```python
from build123d import *

# Parameters (mm, degrees)
F0_R     = 1.651
F1_DEPTH = 3.175
F2_R     = 1.651
F3_DEPTH = 25.4


with BuildPart() as f1:
    # F0 (on Front) → F1 (new body)
    with BuildSketch(Plane.XZ):
        with BuildLine():
            Line((65.389104, 5.08), (65.389104, 0))
            Line((65.389104, 0), (111.109104, 0))
            Line((111.109104, 0), (134.019904, 0))
            Line((134.019904, 0), (139.049104, 0))
            Line((139.049104, 0), (139.477193, 0))
            ThreePointArc((139.477193, 0), (148.009982, 3.664074), (152.4, 11.847085))
            Line((152.4, 11.847085), (152.4, 30.797511))
            ThreePointArc((152.4, 30.797511), (134.859224, 59.672781), (105.392106, 76.2))
            Line((105.392106, 76.2), (37.521991, 76.2))
            Line((37.521991, 76.2), (12.7, 76.2))
            Line((12.7, 76.2), (12.7, 71.12))
            Line((12.7, 71.12), (0, 71.12))
            Line((0, 71.12), (0, 76.2))
            Line((0, 76.2), (-25.4, 76.2))
            Line((-25.4, 76.2), (-25.4, 71.12))
            Line((-25.4, 71.12), (-38.1, 71.12))
            Line((-38.1, 71.12), (-38.1, 76.2))
            Line((-38.1, 76.2), (-50.8, 76.2))
            Line((-50.8, 76.2), (-50.8, 0))
            Line((-50.8, 0), (-19.015096, 0))
            Line((-19.015096, 0), (-19.015096, 5.08))
            Line((-19.015096, 5.08), (65.389104, 5.08))
        make_face()
        with Locations((-36.449, 11.697368)):
            Circle(F0_R, mode=Mode.SUBTRACT)
        with Locations((-12.364374, 17.884336)):
            Circle(F0_R, mode=Mode.SUBTRACT)
        with Locations((16.566699, 25.316282)):
            Circle(F0_R, mode=Mode.SUBTRACT)
        with Locations((40.651325, 31.503251)):
            Circle(F0_R, mode=Mode.SUBTRACT)
        with Locations((79.176886, 41.399872)):
            Circle(F0_R, mode=Mode.SUBTRACT)
        with Locations((104.294765, 47.852268)):
            Circle(F0_R, mode=Mode.SUBTRACT)
    extrude(amount=F1_DEPTH)

    # F2 (on face) → F3 (cut)
    with BuildSketch(Plane.XZ.offset(3.175)):
        with Locations((148.009982, 9.237001)):
            Circle(F2_R)
    extrude(amount=-F3_DEPTH, mode=Mode.SUBTRACT)


solid = f1.part
```
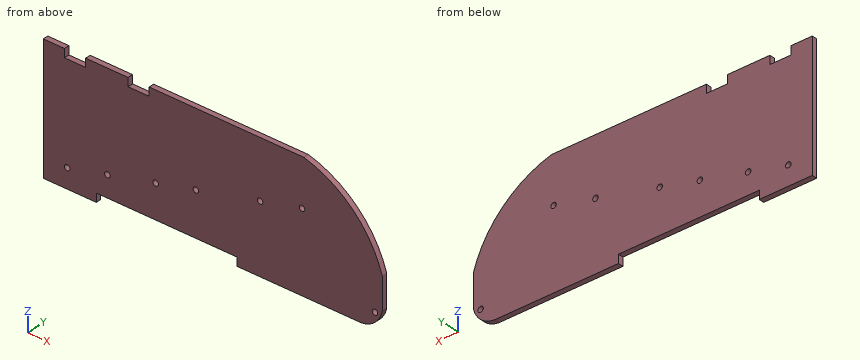
The model under review builds one solid part; all positions refer to its coordinate system, in mm. Coordinates: 2 decimals unless noted, no trailing zeros. Write each loop counter-clockwise with the first axis right and the second up, starting at its lowest first coordinate (ties: lowest second). Pieces come first, ordered by that corner, then holes. Notation, with made-up numbers: (80, 45) - (120, 45) arc R6 ccw to (120, 53) - close; hole circle Ø7 at (42, 43). An arc over 180 degrees is marked (long way). Answer in a Markdown table with one row per item. Add a question column.
Q1. Clearance check with flat-ended pins moving along their axes: pin 1 (1.6 mm diameter, centred on x = 9, y = -2, fed in from +Z); pin 2 (1.6 mm diameter, centred on y = -2, z = 2, fed in from +X). State where each tip first meets the part, or that it passes through.
Q2. Consider section C-C on z = 53.5. Give the boundary of the cut face in (x, y) (3 decimals).
Q3. Consider section B-B on x = 25.5. Give the boundary of the cut face in (y, z) (3 decimals).
Q4. To check wall thickness, follow line 1 along X through (y, z) = (-2.4, 72); line 2 along Z through (x, y) = (63, -2.5); line 3 along Z through (x, y) = (-29, -0.4). State the ranges of each line that lie inside material, in increasing order. Write a range as from..to.
Q5. Consider section A-A on y = -1.95. Give the boundary of the cut face in (x, z), then the cut area to 3 significant figures.
Answers below:
| question | item | result |
|---|---|---|
| 1 | pin 1 | z = 71.12 |
| 1 | pin 2 | x = 146.97 |
| 2 | outline | (-50.8, -3.175) - (140.494, -3.175) - (140.494, 0) - (-50.8, 0) - close |
| 3 | outline | (-3.175, 5.08) - (0, 5.08) - (0, 76.2) - (-3.175, 76.2) - close |
| 4 | line 1 | -50.8..-38.1, -25.4..0, 12.7..117 |
| 4 | line 2 | 5.08..76.2 |
| 4 | line 3 | 0..71.12 |
| 5 | outline | (-50.8, 0) - (-19.02, 0) - (-19.02, 5.08) - (65.39, 5.08) - (65.39, 0) - (139.48, 0) arc R14.07 ccw to (152.4, 11.85) - (152.4, 30.8) arc R66.49 ccw to (105.39, 76.2) - (12.7, 76.2) - (12.7, 71.12) - (0, 71.12) - (0, 76.2) - (-25.4, 76.2) - (-25.4, 71.12) - (-38.1, 71.12) - (-38.1, 76.2) - (-50.8, 76.2) - close; hole circle Ø3.3 at (-36.45, 11.7); hole circle Ø3.3 at (-12.36, 17.88); hole circle Ø3.3 at (16.57, 25.32); hole circle Ø3.3 at (40.65, 31.5); hole circle Ø3.3 at (79.18, 41.4); hole circle Ø3.3 at (104.29, 47.85); hole circle Ø3.3 at (148.01, 9.24) |
| 5 | area | 14,100 mm² |
